```python
from build123d import *

# Parameters (mm, degrees)
SKETCH1_W           = 104.8
SKETCH1_H           = 90
BOSS_EXTRUDE1_DEPTH = 29.7
SKETCH2_W           = 63.5
SKETCH2_H           = 116
BOSS_EXTRUDE2_DEPTH = 2
CUT_EXTRUDE1_DEPTH  = 3
SKETCH4_R           = 1.25
SKETCH4_W           = 9
SKETCH4_H           = 9
SKETCH4_W_2         = 14.5
SKETCH4_H_2         = 16
SKETCH4_W_3         = 6
SKETCH4_H_3         = 14
SKETCH4_W_4         = 16
SKETCH4_H_4         = 13.5
CUT_EXTRUDE2_DEPTH  = 4
CUT_EXTRUDE4_START  = 2
SKETCH5_R           = 1.25
CUT_EXTRUDE4_DEPTH  = 2
SKETCH6_R           = 17.5
SKETCH6_R_2         = 14
CUT_EXTRUDE5_DEPTH  = 1.5
SKETCH7_R           = 12
SKETCH7_R_2         = 8.5
CUT_EXTRUDE6_DEPTH  = 1.5
SKETCH8_R           = 1.6
CUT_EXTRUDE7_DEPTH  = 2
SKETCH9_W           = 90
SKETCH9_H           = 1
CUT_EXTRUDE8_DEPTH  = 0.6
SKETCH10_W          = 90
SKETCH10_H          = 1
CUT_EXTRUDE10_DEPTH = 0.6


with BuildPart() as part:
    # Sketch1 → Boss-Extrude1 (new body)
    with BuildSketch(Plane(origin=(0, 0, 0), x_dir=(1, 0, 0), z_dir=(0, 1, 0))):
        Rectangle(SKETCH1_W, SKETCH1_H)
    extrude(amount=BOSS_EXTRUDE1_DEPTH)

    # Sketch2 → Boss-Extrude2 (add)
    with BuildSketch(Plane(origin=(0, 0, 0), x_dir=(1, 0, 0), z_dir=(0, 1, 0))):
        Rectangle(SKETCH2_W, SKETCH2_H)
    extrude(amount=-BOSS_EXTRUDE2_DEPTH)

    # Sketch3 → Cut-Extrude1 (cut)
    with BuildSketch(Plane.XZ.offset(2)):
        with BuildLine():
            Line((18, 53.75), (26, 53.75))
            ThreePointArc((26, 53.75), (28.25, 51.5), (26, 49.25))
            Line((26, 49.25), (18, 49.25))
            ThreePointArc((18, 49.25), (15.75, 51.5), (18, 53.75))
        make_face()
        with BuildLine():
            Line((-26, 53.75), (-18, 53.75))
            ThreePointArc((-18, 53.75), (-15.75, 51.5), (-18, 49.25))
            Line((-18, 49.25), (-26, 49.25))
            ThreePointArc((-26, 49.25), (-28.25, 51.5), (-26, 53.75))
        make_face()
        with BuildLine():
            Line((18, -49.25), (26, -49.25))
            ThreePointArc((26, -49.25), (28.25, -51.5), (26, -53.75))
            Line((26, -53.75), (18, -53.75))
            ThreePointArc((18, -53.75), (15.75, -51.5), (18, -49.25))
        make_face()
        with BuildLine():
            Line((-26, -49.25), (-18, -49.25))
            ThreePointArc((-18, -49.25), (-15.75, -51.5), (-18, -53.75))
            Line((-18, -53.75), (-26, -53.75))
            ThreePointArc((-26, -53.75), (-28.25, -51.5), (-26, -49.25))
        make_face()
    extrude(amount=-CUT_EXTRUDE1_DEPTH, mode=Mode.SUBTRACT)

    # Sketch4 → Cut-Extrude2 (cut)
    with BuildSketch(Plane.XY.offset(45)):
        with Locations((49.4, 3)):
            Circle(SKETCH4_R)
        with Locations((49.4, 26.7)):
            Circle(SKETCH4_R)
        with Locations((-49.4, 3)):
            Circle(SKETCH4_R)
        with Locations((-49.4, 26.7)):
            Circle(SKETCH4_R)
        with Locations((-42, 14)):
            Rectangle(SKETCH4_W, SKETCH4_H)
        with Locations((-25, 12)):
            Rectangle(SKETCH4_W_2, SKETCH4_H_2)
        with Locations((-8.5, 12)):
            Rectangle(SKETCH4_W_3, SKETCH4_H_3)
        with Locations((3, 12)):
            Rectangle(SKETCH4_W_3, SKETCH4_H_3)
        with Locations((19, 11)):
            Rectangle(SKETCH4_W_4, SKETCH4_H_4)
        with Locations((37, 11)):
            Rectangle(SKETCH4_W_4, SKETCH4_H_4)
    extrude(amount=-CUT_EXTRUDE2_DEPTH, mode=Mode.SUBTRACT)

    # Sketch5 → Cut-Extrude4 (cut)
    with BuildSketch(Plane.XY.offset(-45).offset(CUT_EXTRUDE4_START)):
        with Locations((49.4, 3)):
            Circle(SKETCH5_R)
        with Locations((49.4, 26.7)):
            Circle(SKETCH5_R)
        with Locations((-49.4, 3)):
            Circle(SKETCH5_R)
        with Locations((-49.4, 26.7)):
            Circle(SKETCH5_R)
    extrude(amount=-CUT_EXTRUDE4_DEPTH, mode=Mode.SUBTRACT)

    # Sketch6 → Cut-Extrude5 (cut)
    with BuildSketch(Plane(origin=(0, 29.7, 0), x_dir=(1, 0, 0), z_dir=(0, 1, 0))):
        with Locations(Location((25, 5, 0), (0, 0, 270))):
            Circle(SKETCH6_R)
        with Locations(Location((25, 5, 0), (0, 0, 270))):
            Circle(SKETCH6_R_2, mode=Mode.SUBTRACT)
    extrude(amount=-CUT_EXTRUDE5_DEPTH, mode=Mode.SUBTRACT)

    # Sketch7 → Cut-Extrude6 (cut)
    with BuildSketch(Plane(origin=(0, 29.7, 0), x_dir=(1, 0, 0), z_dir=(0, 1, 0))):
        with Locations(Location((25, 5, 0), (0, 0, 270))):
            Circle(SKETCH7_R)
        with Locations(Location((25, 5, 0), (0, 0, 270))):
            Circle(SKETCH7_R_2, mode=Mode.SUBTRACT)
    extrude(amount=-CUT_EXTRUDE6_DEPTH, mode=Mode.SUBTRACT)

    # Sketch8 → Cut-Extrude7 (cut)
    with BuildSketch(Plane(origin=(0, 29.7, 0), x_dir=(1, 0, 0), z_dir=(0, 1, 0))):
        with Locations(Location((41, -11, 0), (0, 0, 270))):
            Circle(SKETCH8_R)
        with Locations(Location((41, 21, 0), (0, 0, 270))):
            Circle(SKETCH8_R)
        with Locations(Location((9, -11, 0), (0, 0, 270))):
            Circle(SKETCH8_R)
        with Locations(Location((9, 21, 0), (0, 0, 270))):
            Circle(SKETCH8_R)
        with BuildLine():
            Line((-39, -7), (-39, -23))
            ThreePointArc((-39, -23), (-40, -24), (-41, -23))
            Line((-41, -23), (-41, -7))
            ThreePointArc((-41, -7), (-40, -6), (-39, -7))
        make_face()
        with BuildLine():
            Line((-39, 23), (-39, 7))
            ThreePointArc((-39, 7), (-40, 6), (-41, 7))
            Line((-41, 7), (-41, 23))
            ThreePointArc((-41, 23), (-40, 24), (-39, 23))
        make_face()
    extrude(amount=-CUT_EXTRUDE7_DEPTH, mode=Mode.SUBTRACT)

    # Sketch9 → Cut-Extrude8 (cut)
    with BuildSketch(Plane(origin=(52.4, 0, 0), x_dir=(0, 0, -1), z_dir=(1, 0, 0))):
        with Locations((0, 7)):
            Rectangle(SKETCH9_W, SKETCH9_H)
        with Locations((0, 12)):
            Rectangle(SKETCH9_W, SKETCH9_H)
        with Locations((0, 17.7)):
            Rectangle(SKETCH9_W, SKETCH9_H)
        with Locations((0, 22.7)):
            Rectangle(SKETCH9_W, SKETCH9_H)
    extrude(amount=-CUT_EXTRUDE8_DEPTH, mode=Mode.SUBTRACT)

    # Sketch10 → Cut-Extrude10 (cut)
    with BuildSketch(Plane(origin=(-52.4, 0, 0), x_dir=(0, 0, -1), z_dir=(1, 0, 0))):
        with Locations((0, 7)):
            Rectangle(SKETCH10_W, SKETCH10_H)
        with Locations((0, 12)):
            Rectangle(SKETCH10_W, SKETCH10_H)
        with Locations((0, 17.7)):
            Rectangle(SKETCH10_W, SKETCH10_H)
        with Locations((0, 22.7)):
            Rectangle(SKETCH10_W, SKETCH10_H)
    extrude(amount=CUT_EXTRUDE10_DEPTH, mode=Mode.SUBTRACT)


solid = part.part
```
The model under review builds one solid part; all positions refer to its coordinate system, in mm. A direction names the side the tool comes from. Give positions to 0.01 mm unless a question says otherwise; leave off trailing zeros. Write each loop counter-clockwise with the first axis right and the second up, starting at its lowest first coordinate (ties: lowest second). Pieces come first, ordered by that corner, then holes. Notation, with made-up numbers: M 18,84 L 65,84 A18 ccw 65,100 Z; hole C -34,59 d10. An arc over 180 degrees is marked long. Answer in a Markdown table with one row per item.
Item 1: Add section D-D on x = 41. Give the boundary of the cut face in (y, z), plus the area to 3 significant figures.
Check sheet entries:
| item | result |
|---|---|
| outline | M 0,-45 L 29.7,-45 L 29.7,-22.6 L 27.7,-22.6 L 27.7,-19.4 L 29.7,-19.4 L 29.7,-12.09 L 28.2,-12.09 L 28.2,2.09 L 29.7,2.09 L 29.7,9.4 L 27.7,9.4 L 27.7,12.6 L 29.7,12.6 L 29.7,45 L 17.75,45 L 17.75,41 L 4.25,41 L 4.25,45 L 0,45 Z |
| area | 2,580 mm2 |
Item 2: Draft analysis for pull direction Z (two halves, no side actions). For faces 1 (the face through (-49, 3, 41)), 2 (the face through (11.33, 28.96, -8.03)), 3 (the face through (50.59, 3.38, -43.99)), state which applies: +Z half, -Z half, draft (parallel to the pull), parting line (faces both ways), or undercut.
Check sheet entries:
| item | result |
|---|---|
| face 1 | +Z half |
| face 2 | undercut |
| face 3 | draft |
Item 3: Add section A-A on z = 51.5. Give the boundary of the cut face in (x, y).
Check sheet entries:
| item | result |
|---|---|
| outline | M -31.75,-2 L -28.25,-2 L -28.25,0 L -31.75,0 Z; M -15.75,-2 L 15.75,-2 L 15.75,0 L -15.75,0 Z; M 28.25,-2 L 31.75,-2 L 31.75,0 L 28.25,0 Z |
Item 4: Add section C-C on z = -47.5. Give the boundary of the cut face in (x, y), plus the area to 3 significant figures.
Check sheet entries:
| item | result |
|---|---|
| outline | M -31.75,-2 L 31.75,-2 L 31.75,0 L -31.75,0 Z |
| area | 127 mm2 |
Item 5: Add section B-B on x = -44. Give the boundary of the cut face in (y, z), plus the area to 3 significant figures.
Check sheet entries:
| item | result |
|---|---|
| outline | M 0,-45 L 29.7,-45 L 29.7,45 L 18.5,45 L 18.5,41 L 9.5,41 L 9.5,45 L 0,45 Z |
| area | 2,640 mm2 |
Item 6: Tool access review of faces 4 (the face through (42.35, 28.96, -7.28)), 5 (the face through (52.4, 3, 1)), 6 (the face through (11, 11, 43)), 7 (the face through (0, 0, 51)): name each direction out of +Z, -Z, +X, -X, +Y, -Y from which nothing blocks a thin tool from reaching the whole face with its end or side.
Check sheet entries:
| item | result |
|---|---|
| face 4 | +Y |
| face 5 | +Z, -Z, +X, +Y, -Y |
| face 6 | +Z |
| face 7 | +Z, +X, -X, +Y |
Item 7: For P1, Ø2, axis at x = -49.4, y = 3, coming from the +Z side; P2, Ø0.8, axis at x = -49, y = 2.5, coming from the -Z side; P3, Ø5, axis at x = -22.5, y = 24, coming from the -Z side, all flat-tipped, find the tip position at first contact; note any pin that passes through.
Check sheet entries:
| item | result |
|---|---|
| P1 | z = 41 |
| P2 | z = -43 |
| P3 | z = -45 |
Item 8: For line 1 along X through (y, z) = (28.5, 11); line 2 along Y through (x, z) = (-49, 42); line 3 along Z through (x, y) = (32.5, 0.5), list the stretches that pass through material, from the lowest coordinate up.
Check sheet entries:
| item | result |
|---|---|
| line 1 | -52.4 to -41, -39 to 7.4, 10.6 to 17.91, 32.09 to 39.4, 42.6 to 52.4 |
| line 2 | 0 to 1.82, 4.18 to 25.52, 27.88 to 29.7 |
| line 3 | -45 to 45 |
